from build123d import *

# Parameters (mm, degrees)
REVOLVE1_ANGLE     = 40
SKETCH3_R          = 3.2639
CUT_EXTRUDE1_DEPTH = 205.703085759


with BuildPart() as part:
    # Sketch1 → Revolve1 (revolve)
    with BuildSketch(Plane(origin=(0, 0, 0), x_dir=(1, 0, 0), z_dir=(0, 1, 0))):
        Polygon((0, 152.4), (-9.525, 152.4), (-9.525, 171.45), (9.525, 171.45), (9.525, 152.4), align=None)
    revolve(axis=Axis((0, 0, 0), (1, 0, 0)), revolution_arc=REVOLVE1_ANGLE)

    # Sketch2 → Cut-Revolve1 (revolve, cut)
    with BuildSketch(Plane(origin=(0, 0, 0), x_dir=(1, 0, 0), z_dir=(0, 1, 0))):
        with BuildLine():
            Line((-117.856, 38.1), (117.856, 38.1))
            ThreePointArc((117.856, 38.1), (0, 155.956), (-117.856, 38.1))
        make_face()
    revolve(axis=Axis((0, 0, 0), (1, 0, 0)), mode=Mode.SUBTRACT)

    # Sketch3 → Cut-Extrude1 (cut, through all)
    with BuildSketch(Plane(origin=(9.525, 0, 0), x_dir=(0, 0, -1), z_dir=(1, 0, 0))):
        with Locations((162.888028743, 14.250855939)):
            Circle(SKETCH3_R)
        with Locations((153.64936083, 55.923793856)):
            Circle(SKETCH3_R)
        with Locations((133.939742895, 93.785617641)):
            Circle(SKETCH3_R)
    extrude(amount=-CUT_EXTRUDE1_DEPTH, mode=Mode.SUBTRACT)


solid = part.part
The listing builds one solid part. Answer for the finished solid, in the listing's coordinates (mm). Coordinates: 2 decimals unless noted, no trailing zeros. Write each loop counter-clockwise with the first axis right and the second up, starting at its lowest first coordinate (ties: lowest second). Pieces come first, ordered by that corner, then holes. Notation, with made-up numbers: (-1, 49) - (39, 49) arc R10 ccw to (39, 54) - close; hole circle Ø6 at (11.5, 61). An arc over 180 degrees is marked (long way). Answer as CSV lines item,"result".
1. Straight lines are drawn through the part: line 1 (Y direction, x = -2.75, z = -132); line 2 (Y direction, x = -7, z = -156.5); line 3 (Z direction, x = -1, y = 54.5). For each, find the intervals that lie inside material, in ascending order. Write a range as [from, to].
Computed values:
line 1,"y = [83, 91.16], [96.41, 109.41]"
line 2,"y = [0, 54.33], [57.51, 70.02]"
line 3,"z = [-162.56, -156.59], [-150.71, -146.12]"
2. Find section B-B (z = -158). Give the vertices of the cut face in (x, y) (3 decimals).
Computed values:
outline,"(-9.525, 0) - (9.525, 0) - (9.525, 66.567) - (-9.525, 66.567) - close"
3. Determine the mould class of faces 1 (the flat face through (0.133, 105.174, -125.341)), 2 (the cylindrical face through (0.13, 91.8, -131.35)), 3 (the cylindrical face through (0.133, 52.738, -152.942)), 4 (the flat face through (-9.525, 51, -151)) for opening direction Z: +Z half, -Z half, draft (parallel to the pull), parting line (faces both ways), or undercut.
Computed values:
face 1,"+Z half"
face 2,"undercut"
face 3,"undercut"
face 4,"draft"
4. Given P1, Ø4, axis at x = 6.5, z = -126.5, coming from the +Y side; P2, Ø1, axis at x = 0, z = -141.5, coming from the +Y side; P3, Ø4, axis at y = 93.79, z = -133.94, coming from the +X side; P4, Ø3, axis at x = 7, y = 99, coming from the -Z side, each flat-ended and moving along its own axis, determine where each tip first touches the part or whether it passes through.
Computed values:
P1,"stops at y = 107.82"
P2,"stops at y = 97.54"
P3,"passes through"
P4,"stops at z = -141.03"
5. Find section A-A (x = -2.5). Give the number of separate pieces and of enclosed holes in the cut face, plus the area to 3 significant figures.
Computed values:
separate pieces,"1"
enclosed holes,"3"
area,"1,670 mm²"
